from build123d import *

# Parameters (mm, degrees)
SKETCH1_W           = 20
SKETCH1_H           = 6.35
SKETCH1_H_2         = 1.5875
BOSS_EXTRUDE1_DEPTH = 6.35


with BuildPart() as part:
    # Sketch1 → Boss-Extrude1 (new body)
    with BuildSketch(Plane.XY):
        Polygon((0, 20), (0, 0), (30, 0), (50, 0), (70, 0), (90, 0), (110, 0), (130, 0), (150, 0), (170, 0), (200, 0), (200, 20), (193.65, 20), (193.65, 40), (200, 40), (200, 60), (193.65, 60), (193.65, 80), (200, 80), (200, 100), (170, 100), (150, 100), (130, 100), (110, 100), (90, 100), (70, 100), (50, 100), (30, 100), (0, 100), (0, 80), (6.35, 80), (6.35, 60), (0, 60), (0, 40), (6.35, 40), (6.35, 20), align=None)
        with Locations((40, -3.175)):
            Rectangle(SKETCH1_W, SKETCH1_H)
        with Locations((80, -3.175)):
            Rectangle(SKETCH1_W, SKETCH1_H)
        with Locations((120, -3.175)):
            Rectangle(SKETCH1_W, SKETCH1_H)
        with Locations((160, -3.175)):
            Rectangle(SKETCH1_W, SKETCH1_H)
        with Locations((40, 100.79375)):
            Rectangle(SKETCH1_W, SKETCH1_H_2)
        with Locations((80, 100.79375)):
            Rectangle(SKETCH1_W, SKETCH1_H_2)
        with Locations((120, 100.79375)):
            Rectangle(SKETCH1_W, SKETCH1_H_2)
        with Locations((160, 100.79375)):
            Rectangle(SKETCH1_W, SKETCH1_H_2)
    extrude(amount=BOSS_EXTRUDE1_DEPTH)


solid = part.part
Read the model definition and answer for the solid it produces. Units are mm, in the model's axes. A direction names the side the tool comes from. Round coordinates to 2 decimals unless told otherwise and drop trailing zeros. Loops run counter-clockwise (first coordinate to the right, second up) from the corner with the lowest first, then second, coordinate; pieces in that order, holes last.
Q1. Which of the six approach directions +Z, -Z, +X, -X, +Y, -Y give full straight-line access (tool end or side, diameter ignored) to faces 1 (the face through (100, 0, 3)), 2 (the face through (100, 100, 3)), 3 (the face through (3, 60, 3))?
Q2. Consider probe 1 along X at (y, z) = (70, 5.25); probe 2 along Y at (x, z) = (57.5, 2.75). Determine where each line is inside the solid, lowest interval first.
Q3. Section B-B on x = 186 is taken. Write down the section's boundary in (y, z).
Q4. Section A-A on y = 63 is taken. Write down the section's boundary in (x, z).
Q5. Each of these flat-tipped pins is pushed along its axis until it touches: pin 1 (3 mm diameter, centred on x = 1.5, z = 3, fed in from -Y); pin 2 (1.7 mm diameter, centred on y = 101, z = 3, fed in from +X); pin 3 (1.9 mm diameter, centred on x = 186.5, z = 4.5, fed in from +Y). Where does it stop, or does it pass through?
Q6. Determine the mould class of faces 4 (the face through (150, -3, 3)), 5 (the face through (200, 10, 3)), 6 (the face through (80, 101.588, 3)) for opening direction X: released by +X, released by -X, zero draft, split by the parting line, or undercut.
Output:
1. face 1: +Z, -Z, -Y
1. face 2: +Z, -Z, +Y
1. face 3: +Z, -Z, -X
2. probe 1: x = 6.35 to 193.65
2. probe 2: y = 0 to 100
3. outline: (0, 0) - (100, 0) - (100, 6.35) - (0, 6.35) - close
4. outline: (6.35, 0) - (193.65, 0) - (193.65, 6.35) - (6.35, 6.35) - close
5. pin 1: stops at y = 0
5. pin 2: stops at x = 170
5. pin 3: stops at y = 100
6. face 4: undercut
6. face 5: released by +X
6. face 6: zero draft
